Design review of the part built by this model. Coordinates are the model's own, in mm. Face numbers are marked on the shaded views. Give positions to 0.01 mm unless a question says otherwise; leave off trailing zeros. Loops run counter-clockwise (first coordinate to the right, second up) from the corner with the lowest first, then second, coordinate; pieces in that order, holes last. Notation, with made-up numbers: M 3,87.5 L 55,87.5 A18 cw 55,95.5 Z; hole C 7,48 d11. An arc over 180 degrees is marked long. Use CSV: the item, a comma, the result in double quotes.
from build123d import *

# Parameters (mm, degrees)
BOSS_EXTRU_1_DEPTH      = 11
CONG_1_R                = 1
ESQUISSE2_R             = 3.2
ENL_V_MAT_EXTRU_1_DEPTH = 5
ESQUISSE3_R             = 2.05
ENL_V_MAT_EXTRU_2_DEPTH = 100.694533451


with BuildPart() as part:
    # Esquisse1 → Boss.-Extru.1 (new body)
    with BuildSketch(Plane.XY):
        with BuildLine():
            Line((-67, 0), (-45, 0))
            Line((-45, 0), (-45, 65))
            ThreePointArc((-45, 65), (-43.535533906, 68.535533906), (-40, 70))
            Line((-40, 70), (40, 70))
            ThreePointArc((40, 70), (43.535533906, 68.535533906), (45, 65))
            Line((45, 65), (45, 0))
            Line((45, 0), (67, 0))
            Line((67, 0), (67, 3))
            ThreePointArc((67, 3), (66.414213562, 4.414213562), (65, 5))
            Line((65, 5), (55, 5))
            ThreePointArc((55, 5), (51.464466094, 6.464466094), (50, 10))
            Line((50, 10), (50, 73))
            ThreePointArc((50, 73), (48.535533906, 76.535533906), (45, 78))
            Line((45, 78), (-45, 78))
            ThreePointArc((-45, 78), (-48.535533906, 76.535533906), (-50, 73))
            Line((-50, 73), (-50, 10))
            ThreePointArc((-50, 10), (-51.464466094, 6.464466094), (-55, 5))
            Line((-55, 5), (-65, 5))
            ThreePointArc((-65, 5), (-66.414213562, 4.414213562), (-67, 3))
            Line((-67, 3), (-67, 0))
        make_face()
    extrude(amount=BOSS_EXTRU_1_DEPTH)

    # Congé1
    cong_1_edges = [part.edges().sort_by_distance(p)[0] for p in [
        (-66.414213562, 4.414213562, 11),
        (-67, 1.5, 11),
        (-50, 41.5, 0),
        (-48.535533906, 76.535533906, 0),
        (0, 78, 0),
        (48.535533906, 76.535533906, 0),
        (50, 41.5, 0),
        (51.464466094, 6.464466094, 0),
        (60, 5, 0),
        (66.414213562, 4.414213562, 0),
        (67, 1.5, 0),
        (45, 32.5, 0),
        (43.535533906, 68.535533906, 0),
        (0, 70, 0),
        (-43.535533906, 68.535533906, 0),
        (-45, 32.5, 11),
        (-45, 32.5, 0),
        (-67, 1.5, 0),
        (-66.414213562, 4.414213562, 0),
        (-60, 5, 0),
        (-51.464466094, 6.464466094, 0),
        (-43.535533906, 68.535533906, 11),
        (0, 70, 11),
        (43.535533906, 68.535533906, 11),
        (45, 32.5, 11),
        (67, 1.5, 11),
        (-51.464466094, 6.464466094, 11),
        (66.414213562, 4.414213562, 11),
        (60, 5, 11),
        (51.464466094, 6.464466094, 11),
        (50, 41.5, 11),
        (48.535533906, 76.535533906, 11),
        (0, 78, 11),
        (-48.535533906, 76.535533906, 11),
        (-50, 41.5, 11),
        (-60, 5, 11),
    ]]
    fillet(cong_1_edges, radius=CONG_1_R)

    # Esquisse2 → Enlèv. mat.-Extru.1 (cut)
    with BuildSketch(Plane.XZ.offset(-70)):
        with Locations(Location((-33.5, 5.5, 0), (0, 0, 270))):
            Circle(ESQUISSE2_R)
        with Locations(Location((33.5, 5.5, 0), (0, 0, 270))):
            Circle(ESQUISSE2_R)
    extrude(amount=-ENL_V_MAT_EXTRU_1_DEPTH, mode=Mode.SUBTRACT)

    # Esquisse3 → Enlèv. mat.-Extru.2 (cut, through all)
    with BuildSketch(Plane(origin=(0, 5, 0), x_dir=(1, 0, 0), z_dir=(0, 1, 0))):
        with Locations(Location((-60, -5.5, 0), (0, 0, 180))):
            Circle(ESQUISSE3_R)
        with Locations(Location((60, -5.5, 0), (0, 0, 180))):
            Circle(ESQUISSE3_R)
    extrude(amount=-ENL_V_MAT_EXTRU_2_DEPTH, mode=Mode.SUBTRACT)


solid = part.part
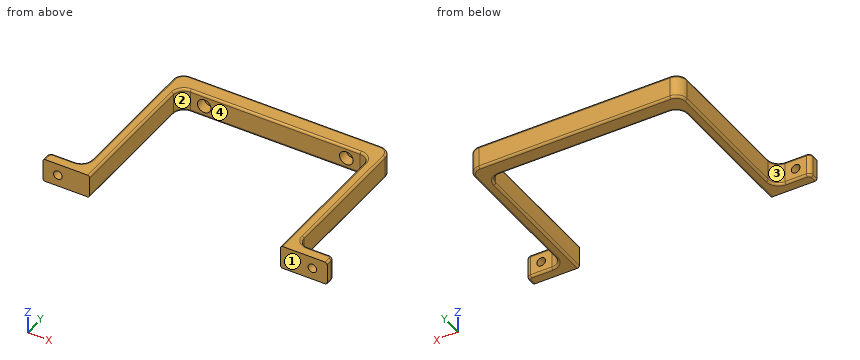
(1) We need section D-D on x = -12. State the section outline as (y, z) points.
A:
outline,"M 70,1 A1 ccw 71,0 L 77,0 A1 ccw 78,1 L 78,10 A1 ccw 77,11 L 71,11 A1 ccw 70,10 Z"
(2) The part is to be moulded in two halves that separate along X. For the marked faces 1, 2, 3 and 4, say which applies: released by +X, released by -X, zero draft, split by the parting line, or undercut.
A:
face 1,"zero draft"
face 2,"undercut"
face 3,"released by -X"
face 4,"undercut"
(3) We need section B-B on y = 19.5. State the section outline as (x, z) points.
A:
outline,"M -50,1 A1 ccw -49,0 L -46,0 A1 ccw -45,1 L -45,10 A1 ccw -46,11 L -49,11 A1 ccw -50,10 Z; M 45,1 A1 ccw 46,0 L 49,0 A1 ccw 50,1 L 50,10 A1 ccw 49,11 L 46,11 A1 ccw 45,10 Z"
(4) We need section C-C on z = 5.5. Count the separate pieces of the cut face and the enclosed holes in it, then the cut area to 3 significant figures.
A:
separate pieces,"3"
enclosed holes,"0"
area,"1,570 mm²"
(5) Wall thickness on line 1 along X through (y, z) = (72.4, 5.5); line 2 along X through (y, z) = (31, 1.5); line 3 along Z through (x, y) = (60, 1.75): over which ranges is each line inside the solid? List them lowest first. Write a range as [from, to].
A:
line 1,"[-50, -36.7], [-30.3, 30.3], [36.7, 50]"
line 2,"[-50, -45], [45, 50]"
line 3,"[0, 3.45], [7.55, 11]"
(6) Clearance check with flat-ended pins moving along their axes: P1, Ø5.5, axis at x = 60, z = 5.5, coming from the -Y side; P2, Ø2.5, axis at y = 56.5, z = 5.5, coming from the +X side; P3, Ø1, axis at x = -19.5, z = 5.5, coming from the -Y side; P4, Ø4.5, axis at x = -61, z = 5.5, coming from the +Y side. State where each tip first meets the part, or that it passes through.
A:
P1,"y = 0"
P2,"x = 50"
P3,"y = 70"
P4,"y = 5"
(7) We need section A-A on x = 60. State the section outline as (y, z) points, then the cut area to 3 significant figures.
A:
outline,"M 0,0 L 4,0 A1 ccw 5,1 L 5,3.45 L 0,3.45 Z; M 0,7.55 L 5,7.55 L 5,10 A1 ccw 4,11 L 0,11 Z"
area,"34.1 mm²"
